Can you work these out from the model? Positions are in its coordinate system, mm. Face numbers are marked on the shaded views. A direction names the side the tool comes from. Give positions to 0.01 mm unless a question says otherwise; leave off trailing zeros. Loops run counter-clockwise (first coordinate to the right, second up) from the corner with the lowest first, then second, coordinate; pieces in that order, holes last. Notation, with made-up numbers: (33, 7) - (43, 7) arc R15 cw to (43, 29) - close; hole circle Ø4 at (-11, 49). An arc over 180 degrees is marked (long way). Answer in a Markdown table with one row per item.
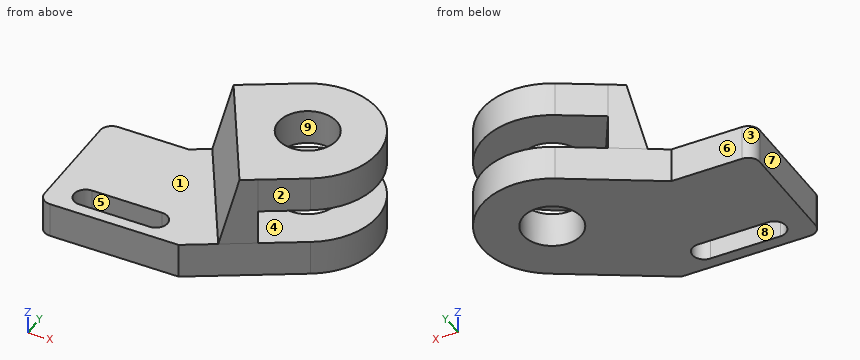
Autodesk Inventor part; units mm, degrees
ref_plane "YZ Plane" through (0, 0, 0) normal (1, 0, 0) x (0, 1, 0)
ref_plane "XZ Plane" through (0, 0, 0) normal (0, 1, 0) x (-1, 0, 0)
ref_plane "XY Plane" through (0, 0, 0) normal (0, 0, 1) x (1, 0, 0)
sketch "Sketch1" plane through (0, 0, 0) normal (0, 0, 1) x (1, 0, 0)
  line L0 (6.35, 0) -> (76.2, 0)
  line L1 (76.2, 0) -> (131.1926, 31.75)
  line L2 (0, 6.35) -> (0, 63.5)
  line L3 (44.7837, 69.85) -> (93.0926, 97.7411)
  arc A0 (131.1926, 31.75) -> (93.0926, 97.7411) centre (112.1426, 64.7456) ccw
  line L4 (6.35, 69.85) -> (44.7837, 69.85)
  circle A1 centre (112.1426, 64.7456) radius 15.875
  arc A2 (6.35, 69.85) -> (0, 63.5) centre (6.35, 63.5) ccw
  arc A3 (0, 6.35) -> (6.35, 0) centre (6.35, 6.35) ccw
  line L5 (19.05, 12.7) -> (57.15, 12.7) construction
  line L6 (19.05, 6.35) -> (57.15, 6.35)
  line L7 (57.15, 19.05) -> (19.05, 19.05)
  arc A4 (19.05, 19.05) -> (19.05, 6.35) centre (19.05, 12.7) ccw
  arc A5 (57.15, 6.35) -> (57.15, 19.05) centre (57.15, 12.7) ccw
  point P0 (0, 0)
  point P1 (0, 69.85)
  point P2 (38.1, 12.7)
  dimension "d0" = 76.2
  dimension "d1" = 69.85
  dimension "d2" = 30
  dimension "d3" = 38.1
  dimension "d4" = 63.5
  dimension "d5" = 31.75
  dimension "d6" = 6.35
  dimension "d7" = 38.1
  dimension "d8" = 12.7
  dimension "d9" = 12.7
  dimension "d10" = 19.05
extrude "Extrusion1" add sketch "Sketch1" along normal blind 19.05
sketch "Sketch2" plane through (131.1926, 31.75, 0) normal (0.5, -0.866, 0) x (0.866, 0.5, 0)
  line L0 (-63.5, 19.05) -> (0, 19.05)
  line L1 (0, 0) -> (-63.5, 0)
  line L2 (-25.4, 19.05) -> (-25.4, 57.15)
  line L3 (-25.4, 57.15) -> (-34.2411, 57.15)
  line L4 (-34.2411, 57.15) -> (-44.45, 19.05)
  point P0 (-129.4911, 0)
  dimension "d16" = 57.15
  dimension "d17" = 75
  dimension "d18" = 19.05
  dimension "d19" = 38.1
extrude "Extrusion2" add sketch "Sketch2" against normal blind 76.2
sketch "Sketch3" plane through (101.5389, 14.6294, 57.15) normal (0, 0, 1) x (0.866, 0.5, 0)
  arc A0 (34.2411, 0) -> (34.2411, 76.2) centre (34.2411, 38.1) ccw
  circle A1 centre (34.2411, 38.1) radius 15.875
  arc A2 (34.2411, 0) -> (34.2411, 76.2) centre (34.2411, 38.1) ccw
  line L0 (8.8411, 76.2) -> (34.2411, 76.2)
  line L1 (34.2411, 0) -> (-29.2589, 0)
  line L2 (8.8411, 0) -> (34.2411, 0)
  line L3 (8.8411, 76.2) -> (8.8411, 0)
  point P0 (-95.25, 38.1)
  dimension "d25" = 31.75
  dimension "d26" = 76.2
extrude "Extrusion3" add sketch "Sketch3" against normal blind 19.05
properties part number "HW 7 Part 2" material "Steel, Carbon"
Q1. Imagine slicing it at A-A, the plane x = 29.5. Write out the boundary of the cut face in (y, z).
Checked values:
| item | result |
|---|---|
| outline | (0, 0) - (6.35, 0) - (6.35, 19.05) - (0, 19.05) - close; (19.05, 0) - (69.85, 0) - (69.85, 19.05) - (19.05, 19.05) - close |
Q2. Imagine slicing it at C-C, the plane x = 52. Write out the boundary of the cut face in (y, z).
Checked values:
| item | result |
|---|---|
| outline | (0, 0) - (6.35, 0) - (6.35, 19.05) - (0, 19.05) - close; (19.05, 0) - (74.02, 0) - (74.02, 19.05) - (19.05, 19.05) - close |
Q3. For pin 1 (8 mm diameter, centred on y = 59, z = 35.5, fed in from +X); pin 2 (9.5 mm diameter, centred on x = 34.5, z = 11.5, fed in from +Y); pin 3 (4 mm diameter, centred on y = 54, z = 19.5, fed in from +X), each with a flat end and sliding along its axis, tell me the tip position at first contact or that it passes through.
Checked values:
| item | result |
|---|---|
| pin 1 | stops at x = 150.15 |
| pin 2 | stops at y = 69.85 |
| pin 3 | stops at x = 149.21 |
Q4. If we mould it in two halves opening along Y, with no side actions, what happens to the marked faces 6, 7, 8 and 9? For each: released by +Y, released by -Y, zero draft, split by the parting line, or undercut.
Checked values:
| item | result |
|---|---|
| face 6 | released by +Y |
| face 7 | zero draft |
| face 8 | undercut |
| face 9 | undercut |
Q5. On a 3-axis mill with a long thin cutter (end or side, diameter ignored), from which of +Z, -Z, +X, -X, +Y, -Y can I reach the whole of each face in a straight line? I mean the marked faces 1, 2, 3, 4 and 5. Say none if no direction works.
Checked values:
| item | result |
|---|---|
| face 1 | +Z, -X, -Y |
| face 2 | +Z, -Z, +X, -Y |
| face 3 | +Z, -Z, -X, +Y |
| face 4 | +X, +Y |
| face 5 | +Z, -Z |
Q6. If I drill on line 1 (Z direction, x = 114.5, y = 35); line 2 (Y direction, x = 44, z = 11.5); line 3 (Z direction, x = 30, y = 62), over which ranges is the centre line in solid material (lowest first)? Write a range as [from, to].
Checked values:
| item | result |
|---|---|
| line 1 | z = [0, 19.05], [38.1, 57.15] |
| line 2 | y = [0, 6.35], [19.05, 69.85] |
| line 3 | z = [0, 19.05] |
Q7. Imagine slicing it at B-B, the plane y = 12.7. Write out the boundary of the cut face in (x, z), and give its area (3 significant figures).
Checked values:
| item | result |
|---|---|
| outline | (0, 0) - (12.7, 0) - (12.7, 19.05) - (0, 19.05) - close; (63.5, 0) - (98.2, 0) - (98.2, 42.75) - (90.86, 19.05) - (63.5, 19.05) - close |
| area | 990 mm² |
Q8. Imagine slicing it at D-D, the plane y = 29. Write out the boundary of the cut face in (x, z), and give its area (3 significant figures).
Checked values:
| item | result |
|---|---|
| outline | (0, 0) - (126.43, 0) - (126.43, 19.05) - (103.45, 19.05) - (103.45, 38.1) - (126.43, 38.1) - (126.43, 57.15) - (93.24, 57.15) - (81.45, 19.05) - (0, 19.05) - close |
| area | 3,460 mm² |
